```python
from build123d import *

# Parameters (mm, degrees)
BOSS_EXTRUDE1_DEPTH = 5
SKETCH2_R           = 5.5
CUT_EXTRUDE1_DEPTH  = 151.352918163
SKETCH3_W           = 40
SKETCH3_H           = 12
BOSS_EXTRUDE2_DEPTH = 5
SKETCH4_R           = 2.1
CUT_EXTRUDE2_DEPTH  = 171.531522013


with BuildPart() as part:
    # Sketch1 → Boss-Extrude1 (new body)
    with BuildSketch(Plane.XY):
        with BuildLine():
            Line((-6.708203932, 6), (-150, 6))
            Line((-150, 6), (-150, -6))
            Line((-150, -6), (-6.708203932, -6))
            ThreePointArc((-6.708203932, -6), (9, 0), (-6.708203932, 6))
        make_face()
    extrude(amount=BOSS_EXTRUDE1_DEPTH)

    # Sketch2 → Cut-Extrude1 (cut, through all)
    with BuildSketch(Plane.XY.offset(5)):
        Circle(SKETCH2_R)
    extrude(amount=-CUT_EXTRUDE1_DEPTH, mode=Mode.SUBTRACT)

    # Sketch3 → Boss-Extrude2 (add)
    with BuildSketch(Plane.XY.offset(5)):
        with Locations((-150, 0)):
            Rectangle(SKETCH3_W, SKETCH3_H)
    extrude(amount=BOSS_EXTRUDE2_DEPTH)

    # Sketch4 → Cut-Extrude2 (cut, through all)
    with BuildSketch(Plane.XY.offset(10)):
        with Locations((-160, 0)):
            Circle(SKETCH4_R)
        with Locations((-140, 0)):
            Circle(SKETCH4_R)
    extrude(amount=-CUT_EXTRUDE2_DEPTH, mode=Mode.SUBTRACT)


solid = part.part
```
Verification items for the finished model (mm, model axes). A direction names the side the tool comes from. Coordinates: 2 decimals unless noted, no trailing zeros. Loops run counter-clockwise (first coordinate to the right, second up) from the corner with the lowest first, then second, coordinate; pieces in that order, holes last. Notation, with made-up numbers: (38, -14.5) -> (63, -14.5) arc R19 cw to (63, 15.5) -> close; hole circle Ø3 at (49, 84). An arc over 180 degrees is marked (long way). Put each result on its own line as item: value.
1. Section check B-B, the plane y = 0. Record the boundary of the cut face in (x, z), then the cut area to 3 significant figures.
Result set:
outline: (-170, 5) -> (-162.1, 5) -> (-162.1, 10) -> (-170, 10) -> close; (-157.9, 5) -> (-150, 5) -> (-150, 0) -> (-142.1, 0) -> (-142.1, 10) -> (-157.9, 10) -> close; (-137.9, 0) -> (-5.5, 0) -> (-5.5, 5) -> (-130, 5) -> (-130, 10) -> (-137.9, 10) -> close; (5.5, 0) -> (9, 0) -> (9, 5) -> (5.5, 5) -> close
area: 877 mm^2
2. Thickness scan on line 1 (Y direction, x = 0, z = 1.35); line 2 (Y direction, x = -140, z = 6.25); line 3 (X direction, y = -1.5, z = 2.5). Record the ranges inside material, lowest first.
Result set:
line 1: y = -9 to -5.5, 5.5 to 9
line 2: y = -6 to -2.1, 2.1 to 6
line 3: x = -150 to -141.47, -138.53 to -5.29, 5.29 to 8.87
3. Gauge pin test, flat ends, axial feed: P1, Ø3, axis at y = 7, z = 7, coming from the -X side; P2, Ø5.5, axis at x = -51.5, y = 0, coming from the +Z side; P3, Ø1, axis at x = -114, y = 7, coming from the +Z side; P4, Ø2.5, axis at y = 3, z = 3.5, coming from the -X side. Record the tip position at first contact, or that the pin passes through.
Result set:
P1: stops at x = -170
P2: stops at z = 5
P3: passes through
P4: stops at x = -150
4. Section check D-D, the plane x = 0. Record the boundary of the cut face in (y, z), then the cut area to 3 significant figures.
Result set:
outline: (-9, 0) -> (-5.5, 0) -> (-5.5, 5) -> (-9, 5) -> close; (5.5, 0) -> (9, 0) -> (9, 5) -> (5.5, 5) -> close
area: 35.0 mm^2
5. Tool access check on faces 1 (the face through (-61, 0, 5)), 2 (the face through (-89, 6, 4)), 3 (the face through (-89, -6, 4)). Record the directions out of +Z, -Z, +X, -X, +Y, -Y that give a thin tool (end or side, any length) a straight path to the whole face; none if there is none.
Result set:
face 1: +Z, +X, +Y, -Y
face 2: +Z, -Z, -X, +Y
face 3: +Z, -Z, -X, -Y
6. Mould release check, pull along Y, two halves, no side actions. Record for faces 4 (the face through (9, 0, 2)), 5 (the face through (-157.997, 0.631, 7.535)), 6 (the face through (-72, 0, 0)): pulls with the +Y half, pulls with the -Y half, needs draft (parallel to the pull), parting line crosses it, or undercut.
Result set:
face 4: parting line crosses it
face 5: undercut
face 6: needs draft
7. Section check C-C, the plane z = 3. Record the boundary of the cut face in (x, y).
Result set:
outline: (-150, -6) -> (-6.71, -6) arc R9 ccw (long way) to (-6.71, 6) -> (-150, 6) -> close; hole circle Ø4.2 at (-140, 0); hole circle Ø11 at (0, 0)
8. Section check A-A, the plane x = -140. Record the boundary of the cut face in (y, z), then the cut area to 3 significant figures.
Result set:
outline: (-6, 0) -> (-2.1, 0) -> (-2.1, 10) -> (-6, 10) -> close; (2.1, 0) -> (6, 0) -> (6, 10) -> (2.1, 10) -> close
area: 78.0 mm^2
